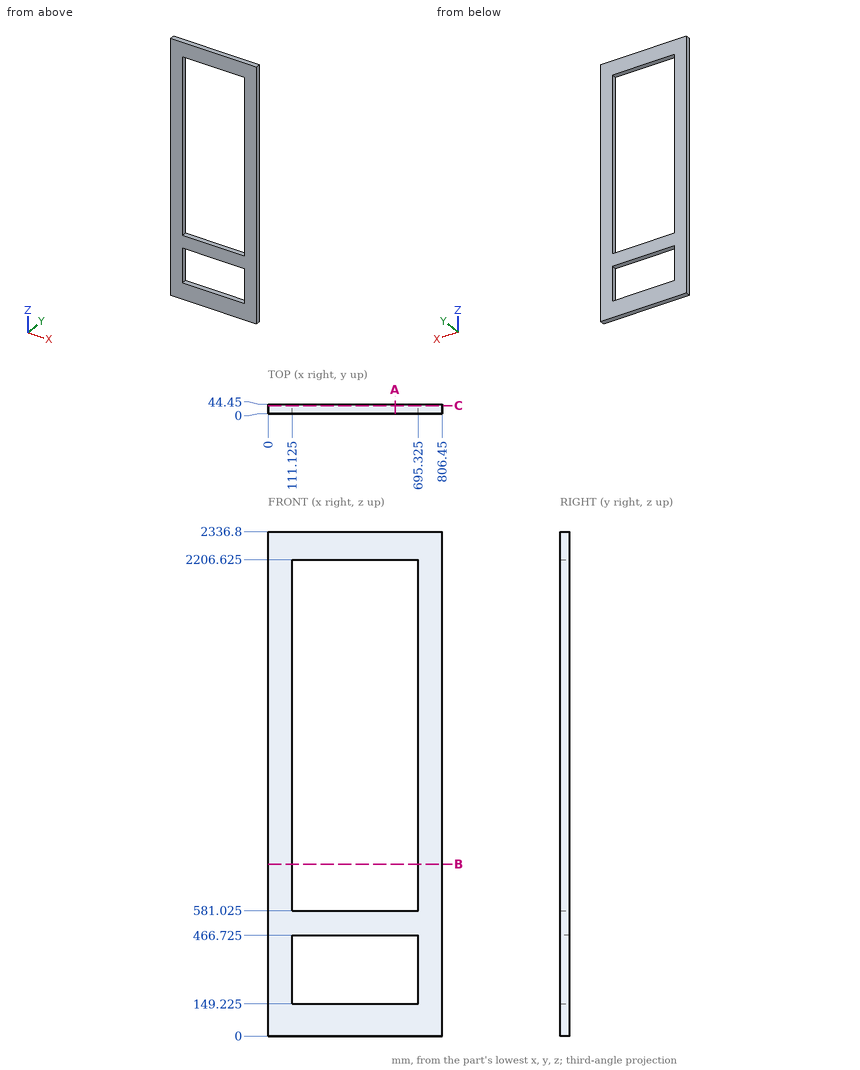
Design review of the part shown in the three views and the two pictorial views. Dimensions are in mm from the part's minimum x, y and z. Coordinates: 2 decimals unless noted, no trailing zeros. Write each loop counter-clockwise with the first axis right and the second up, starting at its lowest first coordinate (ties: lowest second). Pieces come first, ordered by that corner, then holes. Notation, with made-up numbers: (65.5, 62.25) -> (114.5, 62.25) arc R21 ccw to (114.5, 89.25) -> close; hole circle Ø4 at (42.5, 81.25). An arc over 180 degrees is marked (long way). Answer in a Markdown table with one row per item.
1. Wall thickness on probe 1 along Z at (x, y) = (274.5, 28) (3 decimals); probe 2 along X at (y, z) = (24, 233) (3 decimals): over which ranges is each line inside the solid? List them lowest first. Write a range as [from, to].
Answers below:
| item | result |
|---|---|
| probe 1 | z = [0, 149.225], [466.725, 581.025], [2206.625, 2336.8] |
| probe 2 | x = [0, 111.125], [695.325, 806.45] |
2. We need section B-B, the plane z = 796. State the section outline as (x, y) points (3 decimals), and give its area (3 significant figures).
Answers below:
| item | result |
|---|---|
| outline | (0, 0) -> (111.125, 0) -> (111.125, 44.45) -> (0, 44.45) -> close; (695.325, 0) -> (806.45, 0) -> (806.45, 44.45) -> (695.325, 44.45) -> close |
| area | 9,880 mm^2 |
3. We need section A-A, the plane x = 588.5. State the section outline as (y, z) points (3 decimals), and give its area (3 significant figures).
Answers below:
| item | result |
|---|---|
| outline | (0, 0) -> (44.45, 0) -> (44.45, 149.225) -> (0, 149.225) -> close; (0, 466.725) -> (44.45, 466.725) -> (44.45, 581.025) -> (0, 581.025) -> close; (0, 2206.625) -> (44.45, 2206.625) -> (44.45, 2336.8) -> (0, 2336.8) -> close |
| area | 17,500 mm^2 |
4. We need section C-C, the plane y = 36.5. State the section outline as (x, z) points (3 decimals), and give its area (3 significant figures).
Answers below:
| item | result |
|---|---|
| outline | (0, 0) -> (806.45, 0) -> (806.45, 2336.8) -> (0, 2336.8) -> close; hole (111.125, 149.225) -> (695.325, 149.225) -> (695.325, 466.725) -> (111.125, 466.725) -> close; hole (111.125, 581.025) -> (695.325, 581.025) -> (695.325, 2206.625) -> (111.125, 2206.625) -> close |
| area | 749,000 mm^2 |
